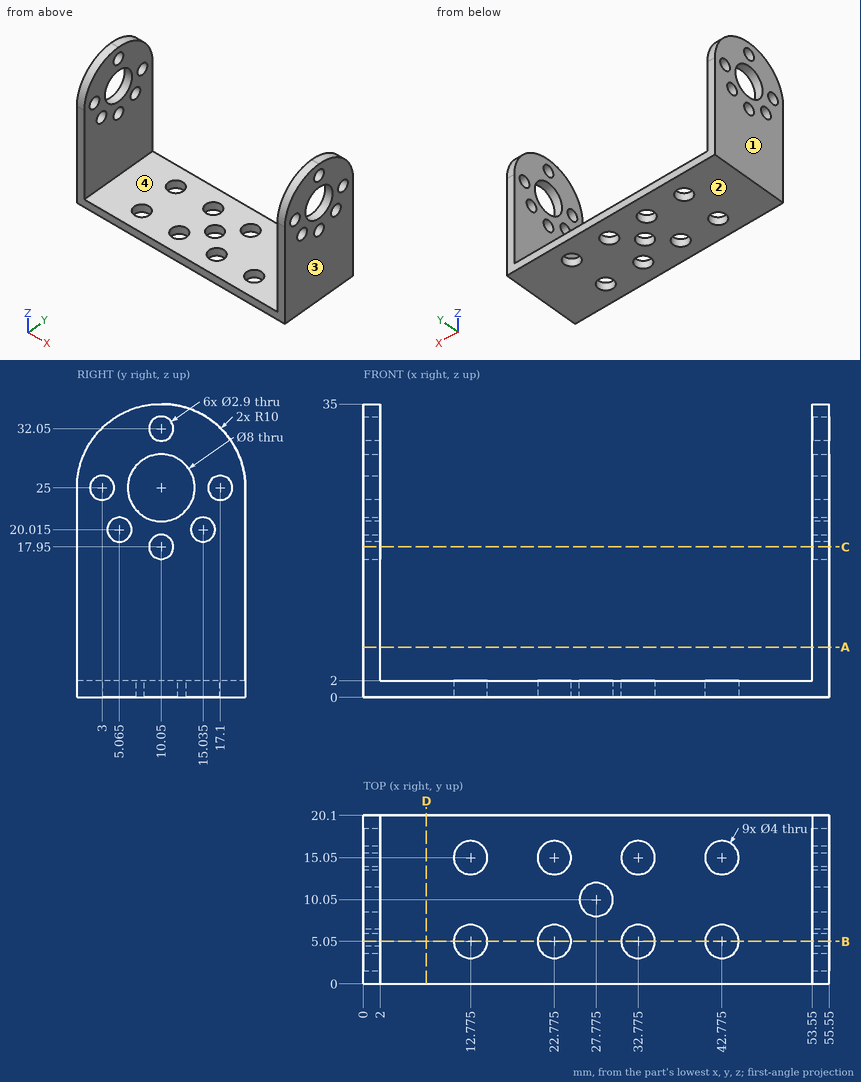
Geometry: see drawing. Coordinates: mm, zero at the bounding-box minimum. Give positions to 0.01 mm unless a question says otherwise; leave off trailing zeros. Order: outer loops, then holes, each group sorted by start corner. A loop starts at its lowest first (then second) coordinate and runs counter-clockwise, first axis right, second up. Notation, with made-up numbers: (41, 74.25) -> (99, 74.25) arc R29 ccw to (99, 108.25) -> close; hole circle Ø2 at (73.25, 62). An arc over 180 degrees is marked (long way). Write each question's results on one line, items separated by ' | '. Start each with the question number.
1) Section D-D (x = 7.5). Return loops of the section in (y, z), then the cut area to 3 significant figures.
2) First-contact query: pin 1 (1 mm diameter, centred on x = 45, y = 18, fed in from +Z); pin 2 (5 mm diameter, centred on y = 10.05, z = 25, fed in from -X). Flat tips, straight axial feed; report the tip coordinate or a pass-through.
3) Section B-B (y = 5.05). Count the separate pieces of the cut face and the enclosed holes in it, then the cut area to 3 significant figures.
4) Line query: line 1 (X direction, y = 5.75, z = 32); line 2 (Z direction, x = 25, y = 10.5); line 3 (Z direction, x = 55.1, y = 3). Output: solid intervals per line, ascending. Write a range as from..to.
5) Draft query along X for the marked faces 1, 2, 3 and 4. Return one class per face: pulls with the +X half, pulls with the -X half, needs draft (parallel to the pull), parting line crosses it, or undercut.
6) Section C-C (z = 17.95). Return loops of the section in (x, y), then the cut area to 3 significant figures.
7) Section A-A (z = 6). Return loops of the section in (x, y), then the cut area to 3 significant figures.
Calculated:
1) outline: (0, 0) -> (20.1, 0) -> (20.1, 2) -> (0, 2) -> close | area: 40.2 mm2
2) pin 1: z = 2 | pin 2: through
3) separate pieces: 7 | enclosed holes: 0 | area: 194 mm2
4) line 1: 0..2, 53.55..55.55 | line 2: 0..2 | line 3: 0..23.55, 26.45..32.14
5) face 1: pulls with the -X half | face 2: needs draft | face 3: pulls with the +X half | face 4: undercut
6) outline: (0, 0) -> (2, 0) -> (2, 8.6) -> (0, 8.6) -> close; (0, 11.5) -> (2, 11.5) -> (2, 20.1) -> (0, 20.1) -> close; (53.55, 0) -> (55.55, 0) -> (55.55, 8.6) -> (53.55, 8.6) -> close; (53.55, 11.5) -> (55.55, 11.5) -> (55.55, 20.1) -> (53.55, 20.1) -> close | area: 68.8 mm2
7) outline: (0, 0) -> (2, 0) -> (2, 20.1) -> (0, 20.1) -> close; (53.55, 0) -> (55.55, 0) -> (55.55, 20.1) -> (53.55, 20.1) -> close | area: 80.4 mm2
